Check sheet for the drawn part. Datum: minimum x, y, z corner. Units: mm. A direction names the side the tool comes from. Round coordinates to 2 decimals unless told otherwise and drop trailing zeros. Write each loop counter-clockwise with the first axis right and the second up, starting at its lowest first coordinate (ties: lowest second). Pieces come first, ordered by that corner, then holes.
Item 1: Material ranges on line 1 (X direction, y = 18, z = 49); line 2 (Z direction, x = 22.5, y = 14); line 3 (Y direction, x = 9, z = 8), recorded low to high.
Item 2: Cross-section at A-A on z = 77.5. Enter the section's corners in (x, y).
Item 3: Tool access check on the marked faces 1, 2, 3, 4 and 5. Record the directions out of +Z, -Z, +X, -X, +Y, -Y that give a thin tool (end or side, any length) a straight path to the whole face; none if there is none.
Item 4: Go/stop test with flat-tipped pins: pin 1 Ø1 at (y, z) = (32.5, 10) entering from +X; pin 2 Ø12 at (x, z) = (25, 31) entering from +Y; pin 3 Ø1 at (x, z) = (14, 40.5) entering from -Y. Record where each tip stops, or that it passes through.
Item 5: Cross-section at D-D on z = 20. Enter the section's corners in (x, y), plus the area to 3 significant figures.
Item 6: Cross-section at B-B on x = 24. Enter the section's corners in (y, z), plus the area to 3 significant figures.
Item 7: Cross-section at C-C on y = 22. Enter the section's corners in (x, z).
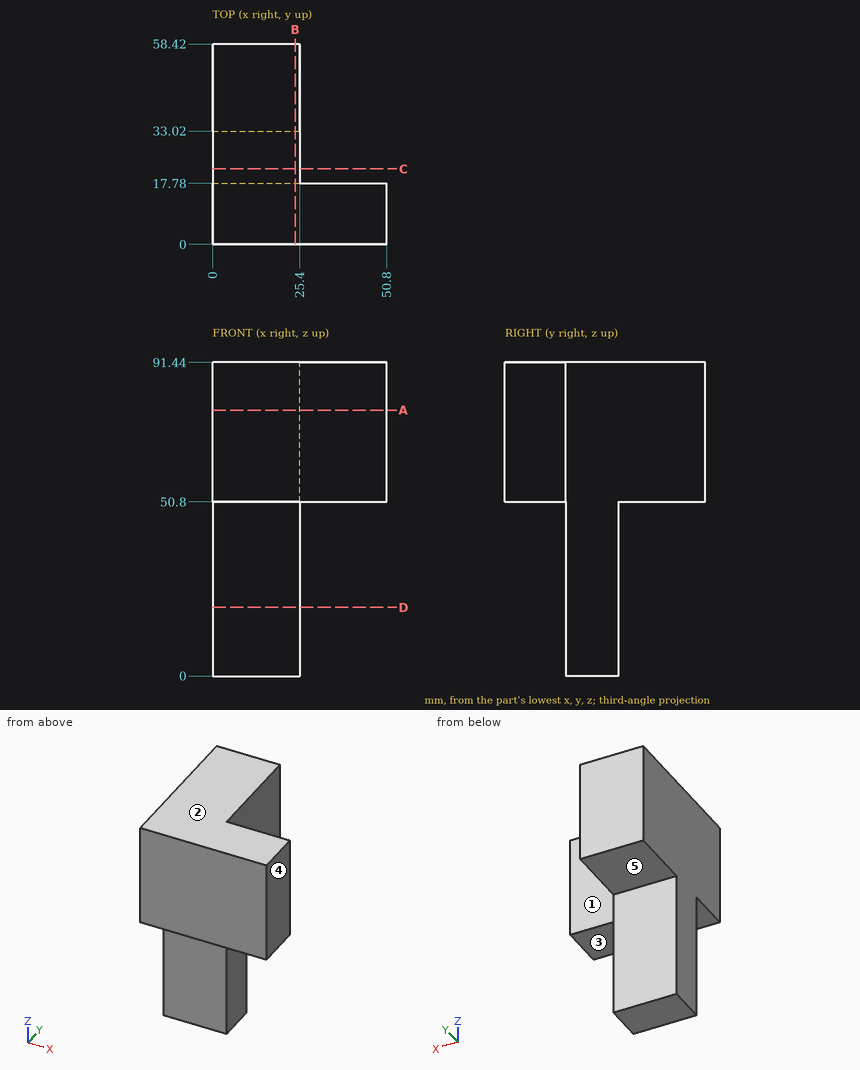
Response values:
1. line 1: x = 0 to 25.4
1. line 2: z = 50.8 to 91.44
1. line 3: y = 17.78 to 33.02
2. outline: (0, 0) - (50.8, 0) - (50.8, 17.78) - (25.4, 17.78) - (25.4, 58.42) - (0, 58.42) - close
3. face 1: +Z, -Z, +X, +Y
3. face 2: +Z, +X, -X, +Y, -Y
3. face 3: -Z, +X, -X, -Y
3. face 4: +Z, -Z, +X, +Y, -Y
3. face 5: -Z, +X, -X, +Y
4. pin 1: stops at x = 25.4
4. pin 2: stops at y = 33.02
4. pin 3: stops at y = 17.78
5. outline: (0, 17.78) - (25.4, 17.78) - (25.4, 33.02) - (0, 33.02) - close
5. area: 387 mm2
6. outline: (0, 50.8) - (17.78, 50.8) - (17.78, 0) - (33.02, 0) - (33.02, 50.8) - (58.42, 50.8) - (58.42, 91.44) - (0, 91.44) - close
6. area: 3,150 mm2
7. outline: (0, 0) - (25.4, 0) - (25.4, 91.44) - (0, 91.44) - close
